Check sheet for the modelled part. Datum: model origin and axes. Units: mm. Face numbers are marked on the shaded views. Round coordinates to 2 decimals unless told otherwise and drop trailing zeros. Write each loop counter-clockwise with the first axis right and the second up, starting at its lowest first coordinate (ties: lowest second). Pieces come first, ordered by that corner, then holes. Notation, with made-up numbers: M 14,45.25 L 57,45.25 A23 ccw 57,76.25 Z; hole C 11,63.5 d4. An arc over 180 degrees is marked long. Answer in a Markdown table with one row per item.
```python
from build123d import *

# Parameters (mm, degrees)
F0_R          = 2.0955
F0_R_2        = 16.8529
F1_DEPTH      = 50.8
F2_R          = 38.1
F3_DEPTH      = 73.152
F3_DEPTH_BACK = 54.61
F4_SIZE       = 1.27
F5_R          = 2.54


with BuildPart() as f1:
    # F0 (on Top) → F1 (new body)
    with BuildSketch(Plane.XY):
        with BuildLine():
            Line((-7.8534178495, 27.3406607066), (-20.1549, 6.35))
            Line((-20.1549, 6.35), (-20.1549, -6.35))
            Line((-20.1549, -6.35), (-7.8534178495, -27.3406607066))
            ThreePointArc((-7.8534178495, -27.3406607066), (-3.0299265704, -30.4461254098), (2.328177165, -28.3965636266))
            Line((2.328177165, -28.3965636266), (20.4851, -8.382))
            Line((20.4851, -8.382), (20.4851, 8.382))
            Line((20.4851, 8.382), (2.328177165, 28.3965636266))
            ThreePointArc((2.328177165, 28.3965636266), (-3.0299265704, 30.4461254098), (-7.8534178495, 27.3406607066))
        make_face()
        with Locations((-2.3749, -24.13)):
            Circle(F0_R, mode=Mode.SUBTRACT)
        Circle(F0_R_2, mode=Mode.SUBTRACT)
        with Locations((-2.3749, 24.13)):
            Circle(F0_R, mode=Mode.SUBTRACT)
    extrude(amount=F1_DEPTH)

    # F2 (on Right) → F3 (cut, two sides)
    with BuildSketch(Plane.YZ) as f3_sk:
        with Locations((0, -12.7)):
            Circle(F2_R)
    extrude(amount=-F3_DEPTH, mode=Mode.SUBTRACT)
    extrude(f3_sk.sketch, amount=F3_DEPTH_BACK, mode=Mode.SUBTRACT)

    # F4
    f4_edges = [f1.edges().sort_by_distance(p)[0] for p in [
        (-16.8529, 0, 50.8),
    ]]
    chamfer(f4_edges, length=F4_SIZE)

    # F5
    f5_edges = [f1.edges().sort_by_distance(p)[0] for p in [
        (20.4851, 8.382, 37.633273),
        (-20.1549, 6.35, 37.833553),
        (-20.1549, -6.35, 37.833553),
        (20.4851, -8.382, 37.633273),
    ]]
    fillet(f5_edges, radius=F5_R)


solid = f1.part
```
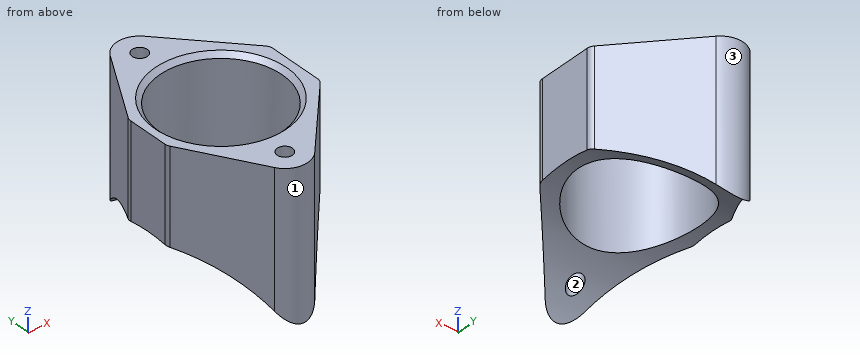
1. Draft check along Y on the marked faces 1, 2 and 3. Enter one of: +Y half, -Y half, draft (parallel to the pull), parting line (faces both ways), or undercut.
Found:
| item | result |
|---|---|
| face 1 | -Y half |
| face 2 | undercut |
| face 3 | +Y half |
2. Section check B-B, the plane y = 0. Record the cut outline in (x, z).
Found:
| item | result |
|---|---|
| outline | M -20.15,25.4 L -16.85,25.4 L -16.85,49.53 L -18.12,50.8 L -20.15,50.8 Z; M 16.85,25.4 L 20.49,25.4 L 20.49,50.8 L 18.12,50.8 L 16.85,49.53 Z |
3. Section check C-C, the plane z = 20.5. Record the cut outline in (x, y).
Found:
| item | result |
|---|---|
| outline | M -12.92,-18.69 L -7.85,-27.34 A6.35 ccw 2.33,-28.4 L 11.13,-18.69 Z; M -12.92,18.69 L 11.13,18.69 L 2.33,28.4 A6.35 ccw -7.85,27.34 Z; hole C -2.37,-24.13 d4.19; hole C -2.37,24.13 d4.19 |
4. Section check A-A, the plane z = 40. Record the cut outline in (x, y), and give its area (3 significant figures).
Found:
| item | result |
|---|---|
| outline | M -20.15,-5.66 A2.54 ccw -19.81,-6.94 L -7.85,-27.34 A6.35 ccw 2.33,-28.4 L 19.83,-9.11 A2.54 ccw 20.49,-7.4 L 20.49,7.4 A2.54 ccw 19.83,9.11 L 2.33,28.4 A6.35 ccw -7.85,27.34 L -19.81,6.94 A2.54 ccw -20.15,5.66 Z; hole C 0,0 d33.71; hole C -2.37,-24.13 d4.19; hole C -2.37,24.13 d4.19 |
| area | 767 mm2 |
5. Scan lines: L1, parallel to X at y = 0, z = 42.75; L2, parallel to X at y = -24, z = 43; L3, parallel to Y at x = -11, z = 42.5. Record each from-to range of solid material in increasing order.
Found:
| item | result |
|---|---|
| L1 | x = -20.15 to -16.85, 16.85 to 20.49 |
| L2 | x = -9.81 to -4.47, -0.28 to 6.32 |
| L3 | y = -21.97 to -12.77, 12.77 to 21.97 |
6. Go/stop test with flat-tipped pins: pin 1 (5 mm diameter, centred on y = 18.5, z = 41, fed in from +X); pin 2 (1 mm diameter, centred on y = 20, z = 25, fed in from +X); pin 3 (3 mm diameter, centred on x = 6, z = 39, fed in from +Y). Record where each tip stops, or that it passes through.
Found:
| item | result |
|---|---|
| pin 1 | stops at x = 13.57 |
| pin 2 | stops at x = 10.4 |
| pin 3 | stops at y = 26 |
7. Section check D-D, the plane y = -25.5. Record the cut outline in (x, z), and give its area (3 significant figures).
Found:
| item | result |
|---|---|
| outline | M -8.93,15.61 L -3.96,15.61 L -3.96,50.8 L -8.93,50.8 Z; M -0.79,15.61 L 4.96,15.61 L 4.96,50.8 L -0.79,50.8 Z |
| area | 377 mm2 |
